Autodesk Inventor part; units mm, degrees
ref_plane "YZ Plane" through (0, 0, 0) normal (1, 0, 0) x (0, 1, 0)
ref_plane "XZ Plane" through (0, 0, 0) normal (0, 1, 0) x (-1, 0, 0)
ref_plane "XY Plane" through (0, 0, 0) normal (0, 0, 1) x (1, 0, 0)
sketch "Sketch1" plane through (0, 0, 0) normal (0, 1, 0) x (-1, 0, 0)
  line L0 (0, 0) -> (0, -20)
  circle A0 centre (0, 0) radius 1.75
  circle A1 centre (0, -20) radius 1.75
  line L1 (0, 0) -> (0, -20) construction
  line L2 (-6, 0) -> (-6, -20)
  line L3 (6, -20) -> (6, 0)
  arc A2 (6, 0) -> (-6, 0) centre (0, 0) ccw
  arc A3 (-6, -20) -> (6, -20) centre (0, -20) ccw
  point P0 (0, -10)
  dimension "d0" = 20
  dimension "d1" = 3.5
  dimension "d2" = 3.5
  dimension "d3" = 12
extrude "Extrusion1" add sketch "Sketch1" along normal blind 1.5
properties part number "LRF Clamp"
Here's how the part is built. I have some questions about the finished solid (model axes, mm). Coordinates: 2 decimals unless noted, no trailing zeros. Loops run counter-clockwise (first coordinate to the right, second up) from the corner with the lowest first, then second, coordinate; pieces in that order, holes last. Notation, with made-up numbers: (36, -24.75) - (86, -24.75) arc R3 cw to (86, -19.75) - close; hole circle Ø11 at (89.25, -30.75). An arc over 180 degrees is marked (long way). Answer as CSV lines item,"result".
Q1. For pin 1 (3 mm diameter, centred on x = 0, z = 0, fed in from -Y), with a flat end and sliding along its axis, tell me the tip position at first contact or that it passes through.
Response:
pin 1,"through"
Q2. If we section it at A-A, the plane x = 0: Write out the boundary of the cut face in (y, z), and give its area (3 significant figures).
Response:
outline,"(0, -26) - (1.5, -26) - (1.5, -21.75) - (0, -21.75) - close; (0, -18.25) - (1.5, -18.25) - (1.5, -1.75) - (0, -1.75) - close; (0, 1.75) - (1.5, 1.75) - (1.5, 6) - (0, 6) - close"
area,"37.5 mm2"
Q3. If I drill on L1, parallel to Z at x = 0, y = 1.1; L2, parallel to Z at x = 1.5, y = 0.3; L3, parallel to X at y = 1.1, z = 0, over which ranges is the centre line in solid material (lowest first)? Write a range as [from, to].
Response:
L1,"[-26, -21.75], [-18.25, -1.75], [1.75, 6]"
L2,"[-25.81, -20.9], [-19.1, -0.9], [0.9, 5.81]"
L3,"[-6, -1.75], [1.75, 6]"
Q4. We'd pull the mould along Z, two halves only. Please class faces 1 (the face through (0, 1, 6)), 2 (the face through (0, 1.5, -10)), 3 (the face through (-1.617, 0.74, 0.67)): pulls with the +Z half, pulls with the -Z half, needs draft (parallel to the pull), parting line crosses it, or undercut.
Response:
face 1,"pulls with the +Z half"
face 2,"needs draft"
face 3,"undercut"
Q5. If we section it at C-C, the plane z = -22.5: Write out the boundary of the cut face in (x, y).
Response:
outline,"(-5.45, 0) - (5.45, 0) - (5.45, 1.5) - (-5.45, 1.5) - close"
Q6. If we section it at D-D, the plane x = -3.5: Write out the boundary of the cut face in (y, z).
Response:
outline,"(0, -24.87) - (1.5, -24.87) - (1.5, 4.87) - (0, 4.87) - close"
Q7. If we section it at B-B, the plane y = 1.1: Write out the boundary of the cut face in (x, z), and give its area (3 significant figures).
Response:
outline,"(-6, -20) arc R6 ccw to (6, -20) - (6, 0) arc R6 ccw to (-6, 0) - close; hole circle Ø3.5 at (0, -20); hole circle Ø3.5 at (0, 0)"
area,"334 mm2"
